The figure shows three views and two pictorial views of one solid part (mm, origin at its lowest corner). Answer the questions. A direction names the side the tool comes from. Round coordinates to 2 decimals unless told otherwise and drop trailing zeros. Loops run counter-clockwise (first coordinate to the right, second up) from the corner with the lowest first, then second, coordinate; pieces in that order, holes last. Notation, with made-up numbers: (6.5, 80.25) -> (45.5, 80.25) arc R31 ccw to (45.5, 112.25) -> close; hole circle Ø10 at (89, 11). An arc over 180 degrees is marked (long way). Put each result on its own line as item: value.
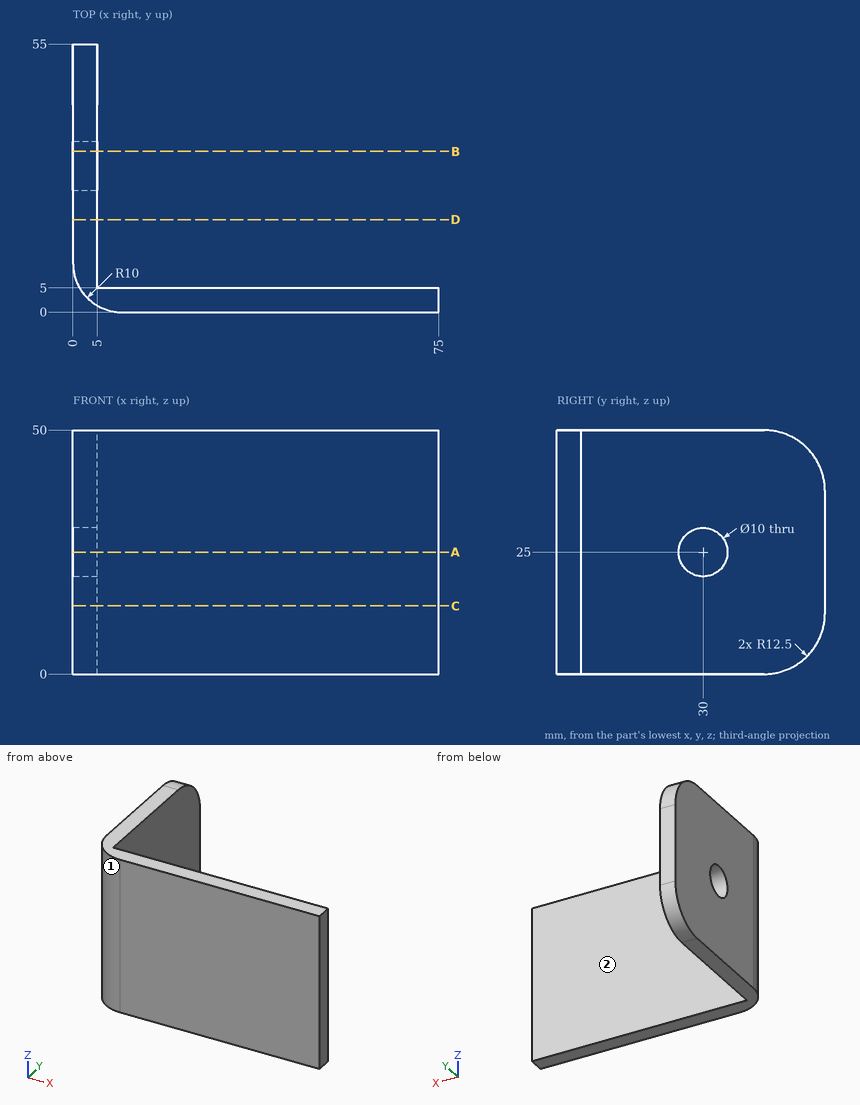
Item 1: The part is cut by section D-D (y = 19). Determine the outline of the cut face in (x, z), then the cut area to 3 significant figures.
Derived:
outline: (0, 0) -> (5, 0) -> (5, 50) -> (0, 50) -> close
area: 250 mm^2
Item 2: Which of the six approach directions +Z, -Z, +X, -X, +Y, -Y give full straight-line access (tool end or side, diameter ignored) to the marked faces 1 and 2?
Derived:
face 1: +Z, -Z, -X, -Y
face 2: +Z, -Z, +X, +Y
Item 3: The part is cut by section A-A (z = 25). Determine the outline of the cut face in (x, y), then the cut area to 3 significant figures.
Derived:
outline: (0, 10) arc R10 ccw to (10, 0) -> (75, 0) -> (75, 5) -> (5, 5) -> (5, 25) -> (0, 25) -> close; (0, 35) -> (5, 35) -> (5, 55) -> (0, 55) -> close
area: 554 mm^2
Item 4: Find the intervals of material crossed by line 1 along Z through (x, y) = (1.5, 30); line 2 along Y through (x, z) = (45, 29.5), in increasing order.
Derived:
line 1: z = 0 to 20, 30 to 50
line 2: y = 0 to 5
Item 5: Flat-ended cylindrical pins translate along their axes: pin 1 Ø15 at (y, z) = (40.5, 19.5) entering from +X; pin 2 Ø6 at (x, z) = (49.5, 36.5) entering from +Y; pin 3 Ø8 at (y, z) = (30, 25) entering from -X. Find the tip coordinate at first contact, or state that the pin passes through.
Derived:
pin 1: stops at x = 5
pin 2: stops at y = 5
pin 3: passes through
Item 6: The part is cut by section B-B (y = 33). Determine the outline of the cut face in (x, z).
Derived:
outline: (0, 0) -> (5, 0) -> (5, 21) -> (0, 21) -> close; (0, 29) -> (5, 29) -> (5, 50) -> (0, 50) -> close
Item 7: The part is cut by section C-C (z = 14). Determine the outline of the cut face in (x, y).
Derived:
outline: (0, 10) arc R10 ccw to (10, 0) -> (75, 0) -> (75, 5) -> (5, 5) -> (5, 55) -> (0, 55) -> close
